```python
from build123d import *

# Parameters (mm, degrees)
SKETCH_R             = 35
SKETCH_R_2           = 6.38
PAD_DEPTH            = 1.2
PAD001_DEPTH         = 1.2
POLARPATTERN_COUNT   = 18
BODY_PLACEMENT_ANGLE = 180


with BuildPart() as part:
    # Sketch → Pad (new body)
    with BuildSketch(Plane.XY):
        Circle(SKETCH_R)
        Circle(SKETCH_R_2, mode=Mode.SUBTRACT)
    extrude(amount=PAD_DEPTH)

    # Sketch001 (on Face4 of Pad) → Pad001 (join)
    with BuildSketch(Plane.XY.offset(1.2)):
        with BuildLine():
            Line((5.56366, 34.554966), (1.372105, 41.147792))
            Line((1.372105, 41.147792), (-6.869961, 42.308363))
            Line((-6.869961, 42.308363), (-3.632167, 37.054228))
            ThreePointArc((-6.589755, 34.374047), (-4.375665, 34.902736), (-3.632167, 37.054228))
            Line((-6.589755, 34.374047), (-4.485629, 26.553919))
            Line((3.9883, 26.28405), (-4.485629, 26.553919))
            Line((5.56366, 34.554966), (3.9883, 26.28405))
        make_face()
    pad001 = extrude(amount=-PAD001_DEPTH)

    # PolarPattern: Pad001 ×18 about axis
    polarpattern_axis = Axis((0, 0, 0), (0, 0, 1))
    for i in range(1, POLARPATTERN_COUNT):
        add(pad001.rotate(polarpattern_axis, i * 360 / POLARPATTERN_COUNT))


with BuildPart() as part_1:
    # Body placement: moved
    add(part.part.moved(Location((0, 0, -2))).rotate(Axis((0, 0, -2), (0, 1, 0)), BODY_PLACEMENT_ANGLE))


solid = part_1.part
```
Geometry check sheet. Reference: the model listing, model coordinates, mm. A direction names the side the tool comes from. Coordinates: 2 decimals unless noted, no trailing zeros. Order: outer loops, then holes, each group sorted by start corner. A loop starts at its lowest first (then second) coordinate and runs counter-clockwise, first axis right, second up.
Q1. Sectioned sample at B-B on y = 4.5. Record the cut outline in (x, z).
Reply:
outline: (-39.35, -3.2) - (-4.52, -3.2) - (-4.52, -2) - (-39.35, -2) - close; (4.52, -3.2) - (41.58, -3.2) - (41.58, -2) - (4.52, -2) - close
Q2. Tool access check on faces 4 (the face through (36.62, 10.01, -2.61)), 5 (the face through (-18.54, -35.52, -2.61)), 6 (the face through (3.5, -37.8, -2.6)), 7 (the face through (-9, -2, -3.2)), 8 (the face through (5.274, 39.718, -2.608)). Record the directions out of +Z, -Z, +X, -X, +Y, -Y that give a thin tool (end or side, any length) a straight path to the whole face; none if there is none.
Reply:
face 4: +Z, -Z, +X
face 5: +Z, -Z, -X
face 6: +Z, -Z, -Y
face 7: -Z, +X, -X, +Y, -Y
face 8: +Z, -Z
Q3. Depth check by flat-ended pin: pin 1 Ø16.5 at (x, y) = (0, 0) entering from -Z. Enter the tip coordinate at first touch or a pass-through.
Reply:
pin 1: stops at z = -3.2
Q4. Draft check along X on faces 1 (the face through (-24.755, 33.689, -2.608)), 2 (the face through (38.2, -12.09, -2.61)), 3 (the face through (11.74, -40.124, -2.608)). Enter one of: released by +X, released by -X, zero draft, split by the parting line, or undercut.
Reply:
face 1: released by -X
face 2: undercut
face 3: released by +X
Q5. Sectioned sample at A-A on x = 0. Record the cut outline in (y, z), and give its area (3 significant figures).
Reply:
outline: (-41.34, -3.2) - (-6.38, -3.2) - (-6.38, -2) - (-41.34, -2) - close; (6.38, -3.2) - (41.34, -3.2) - (41.34, -2) - (6.38, -2) - close
area: 83.9 mm2
Q6. Thickness scan on probe 1 along X at (y, z) = (36, -2.4); probe 2 along X at (y, z) = (35, -2.15); probe 3 along Y at (x, z) = (0, -2.9). Record the ranges inside material, lowest first.
Reply:
probe 1: x = -22.68 to -21.81, -15.85 to -9.25, -4.64 to 3.69, 8.71 to 19.15
probe 2: x = -23.58 to -21.66, -16.07 to -8.77, -5.28 to 4.27, 7.4 to 17.88
probe 3: y = -41.34 to -6.38, 6.38 to 41.34
